For this review, use the dimensioned drawing (mm, ordinates from the lowest corner) and the shaded views. A direction names the side the tool comes from. Give positions to 0.01 mm unless a question says otherwise; leave off trailing zeros. Order: outer loops, then holes, each group sorted by start corner. A loop starts at its lowest first (then second) coordinate and runs counter-clockwise, first axis right, second up. Notation, with made-up numbers: M 52.5,70 L 83.5,70 A27 cw 83.5,103 Z; hole C 26,-22 d10. An arc over 180 degrees is marked long. One line per question, with ' | ' between items. Start each with the question number.
1. The part is to be moulded in two halves that separate along Z. For the marked faces 1, 2 and 3, say which applies: +Z half, -Z half, draft (parallel to the pull), parting line (faces both ways), or undercut.
2. Insertion check: P1, Ø1.4, axis at y = 1.5, z = 5, coming from the -X side; P2, Ø0.9, axis at x = 4.5, z = 5, coming from the -Y side; P3, Ø1, axis at x = 1.5, z = 4.5, coming from the +Y side. Each pin has a flat end and moves straight along its axis. Give the tip position at first contact, or say it passes through.
3. We need section B-B on z = 5. Write out the cut boundary in (x, y).
4. Wall thickness on L1, parallel to Y at x = 5, z = 6.25; L2, parallel to X at y = 7.75, z = 7; L3, parallel to X at y = 3.75, z = 5: over which ranges is each line inside the solid? List them lowest first.
5. For the marked faces 4, 5 and 6, list the 3-axis set-ups (+Z, -Z, +X, -X, +Y, -Y) from which the entire face can be reached by the end or side of a thin tool; tool diameter is ignored.
6. We need section C-C on y = 5. Write out the cut boundary in (x, z), then the cut area to 3 significant figures.
7. We need section A-A on y = 1.25. Write out the cut boundary in (x, z).
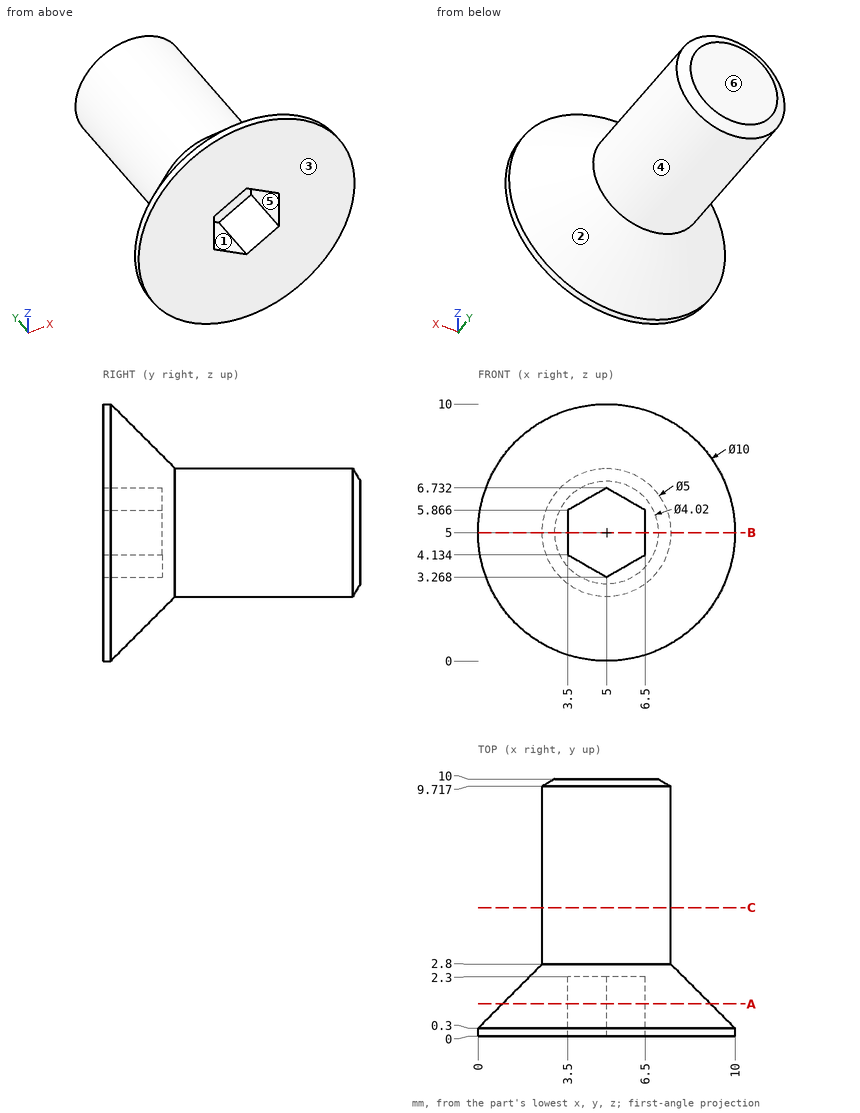
Entries:
1) face 1: undercut | face 2: parting line | face 3: draft
2) P1: stops at x = 0.5 | P2: stops at y = 2.3 | P3: stops at y = 2.26
3) outline: M 0,0 L 3.5,0 L 3.5,2.3 L 6.5,2.3 L 6.5,0 L 10,0 L 10,0.3 L 7.5,2.8 L 7.5,9.72 L 7.01,10 L 2.99,10 L 2.5,9.72 L 2.5,2.8 L 0,0.3 Z
4) L1: y = 2.3 to 10 | L2: x = 3.5 to 6.5 | L3: x = 2.5 to 7.5
5) face 4: +Y | face 5: -Y | face 6: +Z, -Z, +X, -X, +Y
6) outline: C 5,5 d5 | area: 19.6 mm^2
7) outline: C 5,5 d8.1; hole M 3.5,4.13 L 5,3.27 L 6.5,4.13 L 6.5,5.87 L 5,6.73 L 3.5,5.87 Z
